For this review, take the finished solid that the model builds, in its own axes (mm). Coordinates: 2 decimals unless noted, no trailing zeros. Use a Markdown table: item, result.
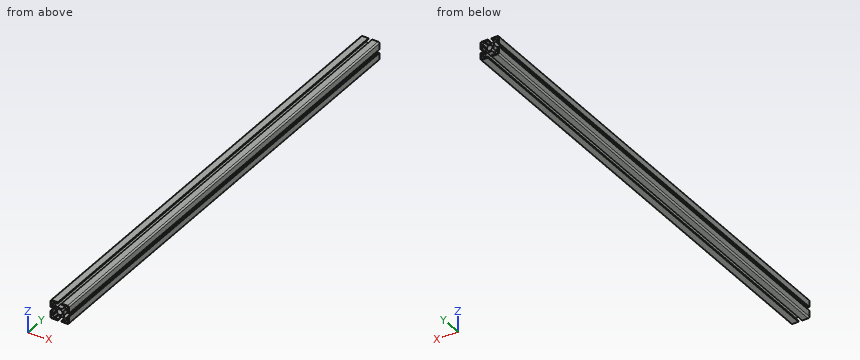
from build123d import *

# Parameters (mm, degrees)
SKETCH1_R           = 6
SKETCH1_R_2         = 3
BOSS_EXTRUDE1_DEPTH = 1050


with BuildPart() as part:
    # Sketch1 → Boss-Extrude1 (new body)
    with BuildSketch(Plane(origin=(0, 0, 0), x_dir=(1, 0, 0), z_dir=(0, 1, 0))):
        with BuildLine():
            Line((-20, -4), (-17, -4))
            Line((-17, -4), (-17, -10))
            Line((-17, -10), (-13, -10))
            Line((-13, -10), (-8.5, -5.5))
            Line((-8.5, -5.5), (-8.5, 5.5))
            Line((-8.5, 5.5), (-13, 10))
            Line((-13, 10), (-17, 10))
            Line((-17, 10), (-17, 4))
            Line((-17, 4), (-20, 4))
            Line((-20, 4), (-20, 17))
            ThreePointArc((-20, 17), (-19.121320344, 19.121320344), (-17, 20))
            Line((-17, 20), (-4, 20))
            Line((-4, 20), (-4, 17))
            Line((-4, 17), (-10, 17))
            Line((-10, 17), (-10, 13))
            Line((-10, 13), (-5.5, 8.5))
            Line((-5.5, 8.5), (5.5, 8.5))
            Line((5.5, 8.5), (10, 13))
            Line((10, 13), (10, 17))
            Line((10, 17), (4, 17))
            Line((4, 17), (4, 20))
            Line((4, 20), (17, 20))
            ThreePointArc((17, 20), (19.121320344, 19.121320344), (20, 17))
            Line((20, 17), (20, 4))
            Line((20, 4), (17, 4))
            Line((17, 4), (17, 10))
            Line((17, 10), (13, 10))
            Line((13, 10), (8.5, 5.5))
            Line((8.5, 5.5), (8.5, -5.5))
            Line((8.5, -5.5), (13, -10))
            Line((13, -10), (17, -10))
            Line((17, -10), (17, -4))
            Line((17, -4), (20, -4))
            Line((20, -4), (20, -17))
            ThreePointArc((20, -17), (19.121320344, -19.121320344), (17, -20))
            Line((17, -20), (4, -20))
            Line((4, -20), (4, -17))
            Line((4, -17), (10, -17))
            Line((10, -17), (10, -13))
            Line((10, -13), (5.5, -8.5))
            Line((5.5, -8.5), (-5.5, -8.5))
            Line((-5.5, -8.5), (-10, -13))
            Line((-10, -13), (-10, -17))
            Line((-10, -17), (-4, -17))
            Line((-4, -17), (-4, -20))
            Line((-4, -20), (-17, -20))
            ThreePointArc((-17, -20), (-19.121320344, -19.121320344), (-20, -17))
            Line((-20, -17), (-20, -4))
        make_face()
        with Locations(Location((0, 0, 0), (0, 0, 270))):
            Circle(SKETCH1_R, mode=Mode.SUBTRACT)
        with Locations(Location((-15, -15, 0), (0, 0, 270))):
            Circle(SKETCH1_R_2, mode=Mode.SUBTRACT)
        with Locations(Location((-15, 15, 0), (0, 0, 90))):
            Circle(SKETCH1_R_2, mode=Mode.SUBTRACT)
        with Locations(Location((15, 15, 0), (0, 0, 270))):
            Circle(SKETCH1_R_2, mode=Mode.SUBTRACT)
        with Locations(Location((15, -15, 0), (0, 0, 90))):
            Circle(SKETCH1_R_2, mode=Mode.SUBTRACT)
    extrude(amount=BOSS_EXTRUDE1_DEPTH)


solid = part.part
(1) For pin 1 Ø3 at (x, z) = (-2.5, 1) entering from -Y; pin 2 Ø2.5 at (y, z) = (466, 19) entering from -X; pin 3 Ø0.9 at (x, y) = (-18.5, 296) entering from -Z, all flat-tipped, find the tip position at first contact; note any pin that passes through.
Found:
| item | result |
|---|---|
| pin 1 | passes through |
| pin 2 | stops at x = -19.9 |
| pin 3 | stops at z = -19.81 |
(2) Take a section at A-A on y = 896. State how many separate pieces and enclosed holes the cut face has, plus the area to 3 significant figures.
Found:
| item | result |
|---|---|
| separate pieces | 1 |
| enclosed holes | 5 |
| area | 671 mm^2 |
(3) For line 1 along Z through (x, y) = (-16, 623); line 2 along X through (y, z) = (398.5, 15); line 3 along X through (y, z) = (81.5, -7), list the stretches that pass through material, from the lowest coordinate up.
Found:
| item | result |
|---|---|
| line 1 | z = -20 to -17.83, -12.17 to -10, 10 to 12.17, 17.83 to 20 |
| line 2 | x = -20 to -18, -12 to -10, 10 to 12, 18 to 20 |
| line 3 | x = -20 to -17, -10 to 10, 17 to 20 |
